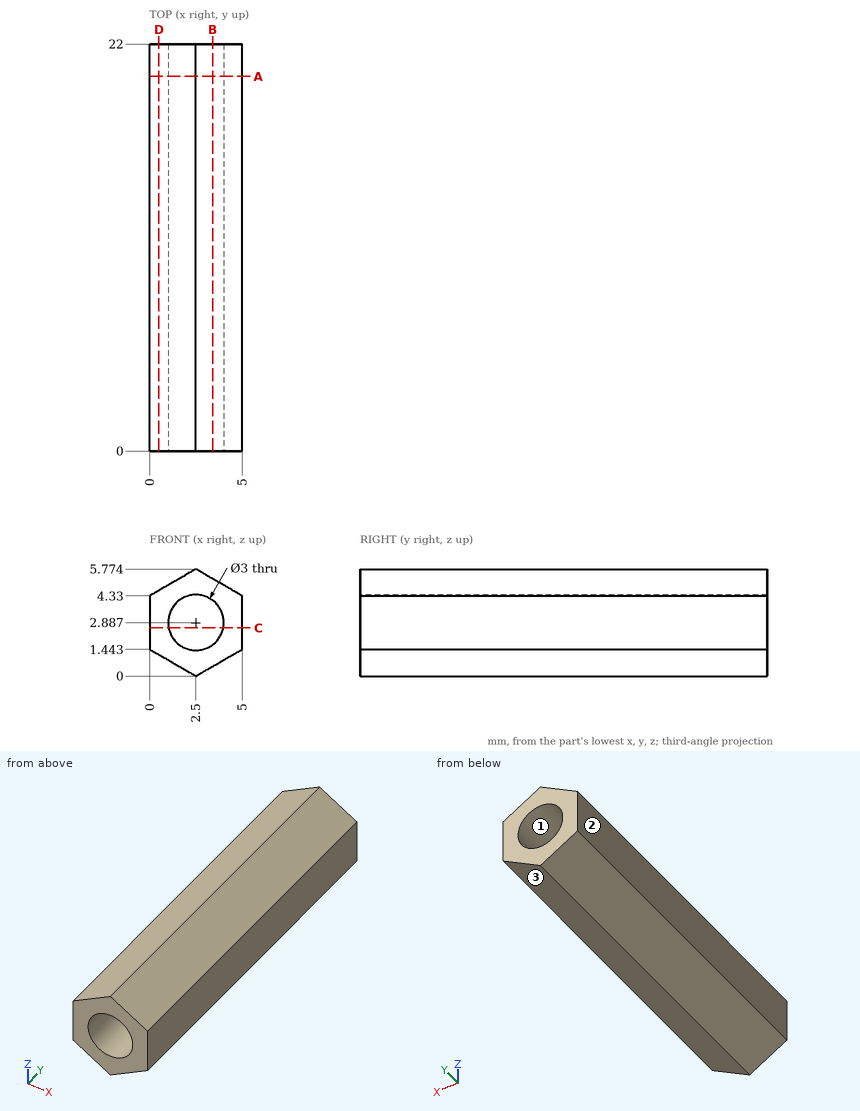
For this review, use the dimensioned drawing (mm, ordinates from the lowest corner) and the shaded views. Coordinates: 2 decimals unless noted, no trailing zeros. Loops run counter-clockwise (first coordinate to the right, second up) from the corner with the lowest first, then second, coordinate; pieces in that order, holes last. Notation, with made-up numbers: (25.25, -5.75) -> (77.25, -5.75) arc R6 ccw to (77.25, -0.75) -> close; hole circle Ø3 at (30, 21.5). An arc over 180 degrees is marked (long way). Return JSON: item names as keys, results as strings. Group by question number.
(1) For pin 1 Ø1.5 at (y, z) = (18.5, 5) entering from -X, flat-tipped, find the tip position at first contact; note if it passes through.
(2) Mouldability with a two-part tool opening along X and no side actions: class the marked faces 1, 2 and 3 as pulls with the +X half, pulls with the -X half, needs draft (parallel to the pull), parting line crosses it, or undercut.
(3) Consider section A-A, the plane y = 20.25. Give the boundary of the cut face in (x, z).
(4) Consider section C-C, the plane z = 2.6. Give the boundary of the cut face in (x, y).
(5) To check wall thickness, follow L1, parallel to Z at x = 3.5, y = 18.5 (1 decimal); L2, parallel to Z at x = 1.4, y = 2.25 (1 decimal); L3, parallel to X at y = 8.25, z = 3.8. State the ranges of each line that lie inside material, in increasing order.
(6) Consider section B-B, the plane x = 3.4. Give the boundary of the cut face in (y, z).
(7) Consider section D-D, the plane x = 0.5. Give the boundary of the cut face in (y, z) (1 decimal).
Results below:
{
 "1": {"pin 1": "stops at x = 0"},
 "2": {"face 1": "undercut", "face 2": "pulls with the -X half", "face 3": "pulls with the +X half"},
 "3": {"outline": "(0, 1.44) -> (2.5, 0) -> (5, 1.44) -> (5, 4.33) -> (2.5, 5.77) -> (0, 4.33) -> close; hole circle Ø3 at (2.5, 2.89)"},
 "4": {"outline": "(0, 0) -> (1.03, 0) -> (1.03, 22) -> (0, 22) -> close; (3.97, 0) -> (5, 0) -> (5, 22) -> (3.97, 22) -> close"},
 "5": {"L1": "z = 0.6 to 1.8, 4 to 5.2", "L2": "z = 0.6 to 1.9, 3.9 to 5.1", "L3": "x = 0 to 1.31, 3.69 to 5"},
 "6": {"outline": "(0, 0.52) -> (22, 0.52) -> (22, 1.69) -> (0, 1.69) -> close; (0, 4.09) -> (22, 4.09) -> (22, 5.25) -> (0, 5.25) -> close"},
 "7": {"outline": "(0, 1.2) -> (22, 1.2) -> (22, 4.6) -> (0, 4.6) -> close"}
}
